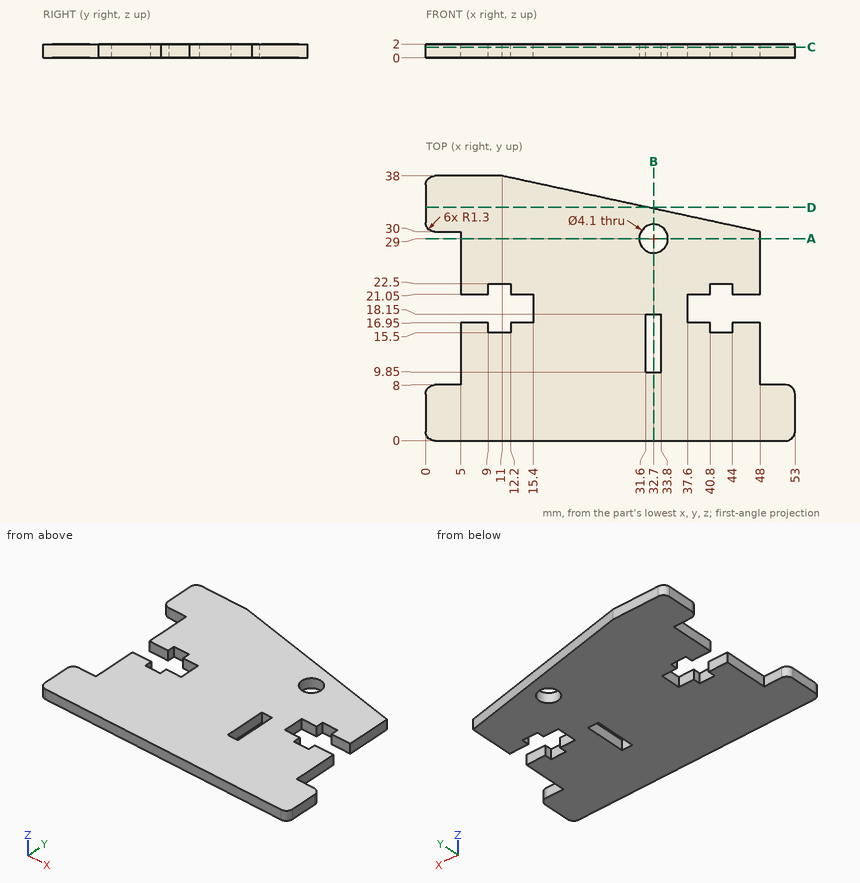
Geometry: see drawing. Coordinates: mm, zero at the bounding-box minimum. Round coordinates to 2 decimals unless told otherwise and drop trailing zeros. Loops run counter-clockwise (first coordinate to the right, second up) from the corner with the lowest first, then second, coordinate; pieces in that order, holes last. Notation, with made-up numbers: (53, 34) -> (99, 34) arc R29 cw to (99, 72) -> close; hole circle Ø2 at (7, 66). An arc over 180 degrees is marked (long way). Write each question's results on one line, items separated by ' | '.
Item 1: Cut plane C-C on z = 1.55. State how many separate pieces and enclosed holes the cut face has, and give its area (3 significant figures).
Answers below:
separate pieces: 1 | enclosed holes: 2 | area: 1,470 mm²
Item 2: Line query: probe 1 along Y at (x, z) = (32.7, 1.4); probe 2 along X at (y, z) = (17.5, 1.35); probe 3 along Y at (x, z) = (31.5, 0.8). Output: solid intervals per line, ascending. Write a range as [from, to].
Answers below:
probe 1: y = [0, 9.85], [18.15, 26.95], [31.05, 33.31] | probe 2: x = [15.4, 31.6], [33.8, 37.6] | probe 3: y = [0, 27.34], [30.66, 33.57]
Item 3: Cut plane B-B on x = 32.7. Return the cut outline in (y, z).
Answers below:
outline: (0, 0) -> (9.85, 0) -> (9.85, 2) -> (0, 2) -> close; (18.15, 0) -> (26.95, 0) -> (26.95, 2) -> (18.15, 2) -> close; (31.05, 0) -> (33.31, 0) -> (33.31, 2) -> (31.05, 2) -> close
Item 4: Pin query (flat end, axial travel): pin 1 Ø0.7 at (y, z) = (21.5, 1) entering from +X; pin 2 Ø1 at (y, z) = (27, 1.5) entering from -X; pin 3 Ø1 at (x, z) = (50.5, 1) entering from +Y. Return the tip coordinate at first contact, or that it passes through.
Answers below:
pin 1: stops at x = 48 | pin 2: stops at x = 5 | pin 3: stops at y = 8
Item 5: Cut plane A-A on y = 29. Return the cut outline in (x, z).
Answers below:
outline: (5, 0) -> (30.65, 0) -> (30.65, 2) -> (5, 2) -> close; (34.75, 0) -> (48, 0) -> (48, 2) -> (34.75, 2) -> close
Item 6: Cut plane D-D on y = 33.5. Return the cut outline in (x, z), and give its area (3 significant figures).
Answers below:
outline: (0, 0) -> (31.81, 0) -> (31.81, 2) -> (0, 2) -> close | area: 63.6 mm²
